Could you check a few things on this model? Use its own coordinates, in mm. Give positions to 0.01 mm unless a question says otherwise; leave off trailing zeros. Loops run counter-clockwise (first coordinate to the right, second up) from the corner with the lowest first, then second, coordinate; pieces in that order, holes last. Notation, with made-up numbers: (73.5, 0.5) - (115.5, 0.5) arc R24 ccw to (115.5, 18.5) - close; hole circle Ø6 at (-38.75, 83.25). An arc over 180 degrees is marked (long way). Answer in a Markdown table with one row per item. Add a question column.
Autodesk Inventor part; units mm, degrees
ref_plane "Work Plane1" through (0, 13, 0) normal (0, 1, 0) x (-1, 0, 0)
ref_plane "YZ Plane" through (0, 0, 0) normal (1, 0, 0) x (0, 1, 0)
ref_plane "XY Plane" through (0, 0, 0) normal (0, 0, 1) x (1, 0, 0)
ref_plane "Work Plane1" through (0, 13, 0) normal (0, 1, 0) x (-1, 0, 0)
sketch "Sketch1" plane through (0, 13, 0) normal (0, 1, 0) x (-1, 0, 0)
  line L0 (5, 6) -> (5, 0)
  line L1 (-5, 6) -> (5, 6)
  line L2 (-5, 0) -> (5, 0)
  line L3 (-5, 6) -> (-5, 0)
extrude "Extrusion1" add sketch "Sketch1" against normal blind 26
hole "Hole2" at (0, -8, 0) direction (0, 0, 1) diameter 4.5 depth 6
sketch "Sketch2" plane through (0, 0, 0) normal (0, 0, 1) x (1, 0, 0)
  point P0 (0, -8)
hole "Hole1" at (0, 8, 0) direction (0, 0, 1) diameter 4.5 depth 6
sketch "Sketch3" plane through (0, 0, 0) normal (0, 0, 1) x (1, 0, 0)
  point P0 (0, 8)
properties part number "carriage Belt clamp" material "ASA Plastic"
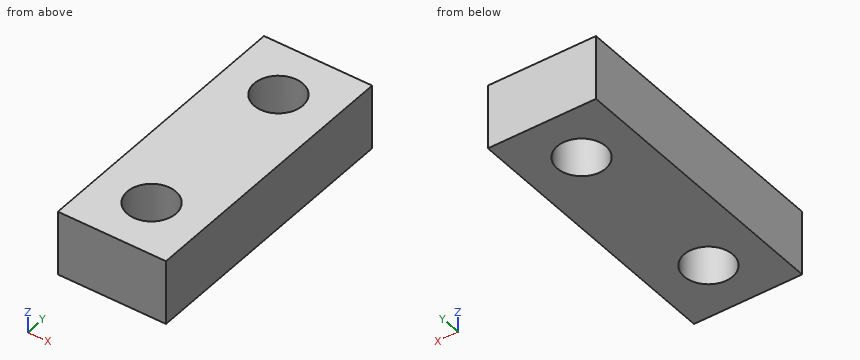
(1) I want a section at B-B on x = 0. Please give me the cut outline in (y, z), then the cut area to 3 significant figures.
(2) For pin 1 Ø4 at (x, y) = (0, -8) entering from +Z, with a flat end and sliding along its axis, tell me the tip position at first contact or that it passes through.
(3) I want a section at A-A on y = -8. Please give me the cut outline in (x, z), then the cut area to 3 significant figures.
(4) I want a section at D-D on y = 9.5. Please give me the cut outline in (x, z), then the cut area to 3 significant figures.
(5) Please list where these lines run through material, in increasing order: line 1 (Y direction, x = 0, z = 4.1); line 2 (X direction, y = 8, z = 4.7); line 3 (Y direction, x = 2, z = 3.35).
(6) I want a section at C-C on z = 5. Please give me the cut outline in (x, y).
Reported:
| question | item | result |
|---|---|---|
| 1 | outline | (-13, 0) - (-10.25, 0) - (-10.25, 6) - (-13, 6) - close; (-5.75, 0) - (5.75, 0) - (5.75, 6) - (-5.75, 6) - close; (10.25, 0) - (13, 0) - (13, 6) - (10.25, 6) - close |
| 1 | area | 102 mm² |
| 2 | pin 1 | through |
| 3 | outline | (-5, 0) - (-2.25, 0) - (-2.25, 6) - (-5, 6) - close; (2.25, 0) - (5, 0) - (5, 6) - (2.25, 6) - close |
| 3 | area | 33.0 mm² |
| 4 | outline | (-5, 0) - (-1.68, 0) - (-1.68, 6) - (-5, 6) - close; (1.68, 0) - (5, 0) - (5, 6) - (1.68, 6) - close |
| 4 | area | 39.9 mm² |
| 5 | line 1 | -13 to -10.25, -5.75 to 5.75, 10.25 to 13 |
| 5 | line 2 | -5 to -2.25, 2.25 to 5 |
| 5 | line 3 | -13 to -9.03, -6.97 to 6.97, 9.03 to 13 |
| 6 | outline | (-5, -13) - (5, -13) - (5, 13) - (-5, 13) - close; hole circle Ø4.5 at (0, -8); hole circle Ø4.5 at (0, 8) |
